```python
from build123d import *

# Parameters (mm, degrees)
SKETCH_1_W      = 24
SKETCH_1_H      = 25
SKETCH_1_R      = 1
EXTRUDE_1_DEPTH = 2
SKETCH_2_R      = 5
EXTRUDE_2_DEPTH = 10


with BuildPart() as part:
    # 草图1 → 凸台-拉伸1 (new body)
    with BuildSketch(Plane.XY):
        with Locations((-12, 12.5)):
            Rectangle(SKETCH_1_W, SKETCH_1_H)
        with Locations((-22.5, 23.5)):
            Circle(SKETCH_1_R, mode=Mode.SUBTRACT)
        with Locations((-22.5, 10.5)):
            Circle(SKETCH_1_R, mode=Mode.SUBTRACT)
        with Locations((-1.5, 10.5)):
            Circle(SKETCH_1_R, mode=Mode.SUBTRACT)
        with Locations((-1.5, 23.5)):
            Circle(SKETCH_1_R, mode=Mode.SUBTRACT)
    extrude(amount=EXTRUDE_1_DEPTH)

    # 草图2 → 凸台-拉伸2 (add)
    with BuildSketch(Plane.XY.offset(2)):
        with Locations((-12, 17)):
            Circle(SKETCH_2_R)
    extrude(amount=EXTRUDE_2_DEPTH)


solid = part.part
```
Work out the finished part from the listing and answer in its coordinate system (mm). A direction names the side the tool comes from. Give positions to 0.01 mm unless a question says otherwise; leave off trailing zeros. Order: outer loops, then holes, each group sorted by start corner. A loop starts at its lowest first (then second) coordinate and runs counter-clockwise, first axis right, second up.
1. Section A-A, the plane x = -1.5 is taken. Determine the outline of the cut face in (y, z).
Result sheet:
outline: (0, 0) - (9.5, 0) - (9.5, 2) - (0, 2) - close; (11.5, 0) - (22.5, 0) - (22.5, 2) - (11.5, 2) - close; (24.5, 0) - (25, 0) - (25, 2) - (24.5, 2) - close
2. Section B-B, the plane y = 10.5 is taken. Determine the outline of the cut face in (x, z), and give its area (3 significant figures).
Result sheet:
outline: (-24, 0) - (-23.5, 0) - (-23.5, 2) - (-24, 2) - close; (-21.5, 0) - (-2.5, 0) - (-2.5, 2) - (-21.5, 2) - close; (-0.5, 0) - (0, 0) - (0, 2) - (-0.5, 2) - close
area: 40.0 mm2
3. Section D-D, the plane x = -12 is taken. Determine the outline of the cut face in (y, z).
Result sheet:
outline: (0, 0) - (25, 0) - (25, 2) - (22, 2) - (22, 12) - (12, 12) - (12, 2) - (0, 2) - close
4. Each of these flat-tipped pins is pushed along its axis until it touches: P1, Ø3, axis at x = -1.5, y = 23.5, coming from the +Z side; P2, Ø1.5, axis at y = 19, z = 9, coming from the -X side; P3, Ø1.6, axis at x = -22.5, y = 10.5, coming from the +Z side; P4, Ø4, axis at y = 11.5, z = 6.5, coming from the -X side. Where does it stop, or does it pass through?
Result sheet:
P1: stops at z = 2
P2: stops at x = -16.84
P3: passes through
P4: stops at x = -15.57
5. For faces 1 (the flat face through (-12, 25, 1)), 2 (the cylindrical face through (-9.693, 12.564, 6.93)), determine the directions among +Z, -Z, +X, -X, +Y, -Y from which every point of the face is accessible in a straight line to the end or side of a thin tool.
Result sheet:
face 1: +Z, -Z, +X, -X, +Y
face 2: +Z
6. Section C-C, the plane y = 17 is taken. Determine the outline of the cut face in (x, z), and give its area (3 significant figures).
Result sheet:
outline: (-24, 0) - (0, 0) - (0, 2) - (-7, 2) - (-7, 12) - (-17, 12) - (-17, 2) - (-24, 2) - close
area: 148 mm2
7. Straight lines are drawn through the part: L1, parallel to Y at x = -22.5, z = 0.65; L2, parallel to Z at x = -20.5, y = 6.25; L3, parallel to X at y = 13.75, z = 5.25. For each, find the intervals that lie inside material, in ascending order.
Result sheet:
L1: y = 0 to 9.5, 11.5 to 22.5, 24.5 to 25
L2: z = 0 to 2
L3: x = -15.8 to -8.2
8. The mould has two halves that part along X. Classify faces 3 (the flat face through (-12, 17, 12)), 4 (the cylindrical face through (-1.63, 11.49, 0.99)), 5 (the flat face through (-24, 12, 1)): released by +X, released by -X, zero draft, split by the parting line, or undercut.
Result sheet:
face 3: zero draft
face 4: undercut
face 5: released by -X
